Autodesk Inventor part; units mm, degrees
ref_plane "YZ Plane" through (0, 0, 0) normal (1, 0, 0) x (0, 1, 0)
ref_plane "XZ Plane" through (0, 0, 0) normal (0, 1, 0) x (-1, 0, 0)
ref_plane "XY Plane" through (0, 0, 0) normal (0, 0, 1) x (1, 0, 0)
sketch "Sketch1" plane through (0, 0, 0) normal (0, 0, 1) x (1, 0, 0)
  line L0 (0, 0) -> (120, 0)
  line L1 (120, 0) -> (120, 80)
  line L2 (120, 80) -> (0, 80)
  line L3 (0, 80) -> (0, 0)
  dimension "d0" = 120
  dimension "d1" = 80
extrude "Extrusion1" add sketch "Sketch1" along normal blind 6
sketch "Sketch2" plane through (0, 0, 6) normal (0, 0, 1) x (1, 0, 0)
  line L0 (0, 0) -> (120, 0)
  line L1 (120, 0) -> (120, 80)
  line L2 (120, 80) -> (0, 80)
  line L3 (0, 80) -> (0, 0)
  line L4 (120, 0) -> (105.25, 0)
  line L5 (105.25, 0) -> (105.25, 6)
  line L6 (105.25, 6) -> (120, 6)
  line L7 (120, 6) -> (120, 0)
  line L8 (0, 0) -> (120, 0)
  line L9 (74.75, 0) -> (45.25, 0)
  line L10 (45.25, 0) -> (45.25, 6)
  line L11 (45.25, 6) -> (74.75, 6)
  line L12 (74.75, 6) -> (74.75, 0)
  line L13 (14.75, 0) -> (0, 0)
  line L14 (0, 0) -> (0, 6)
  line L15 (0, 6) -> (14.75, 6)
  line L16 (14.75, 6) -> (14.75, 0)
  line L17 (120, 80) -> (105.25, 80)
  line L18 (105.25, 80) -> (105.25, 74)
  line L19 (105.25, 74) -> (120, 74)
  line L20 (120, 74) -> (120, 80)
  line L21 (120, 80) -> (0, 80)
  line L22 (74.75, 80) -> (45.25, 80)
  line L23 (45.25, 80) -> (45.25, 74)
  line L24 (45.25, 74) -> (74.75, 74)
  line L25 (74.75, 74) -> (74.75, 80)
  line L26 (14.75, 80) -> (0, 80)
  line L27 (0, 80) -> (0, 74)
  line L28 (0, 74) -> (14.75, 74)
  line L29 (14.75, 74) -> (14.75, 80)
  line L30 (60, -24.5918) -> (60, 107.6161)
  line L31 (0, 80) -> (0, 0)
  dimension "d4" = 6
  dimension "d5" = 6
  dimension "d6" = 14.75
  dimension "d7" = 14.75
  dimension "d8" = 29.5
  dimension "d18" = 60
  dimension "d19" = 14.75
extrude "Extrusion2" cut sketch "Sketch2" against normal up to next contours L3 L15 L16 L0 | L10 L11 L30 L0 | L3 L2 L29 L28 | L30 L11 L12 L0 | L5 L6 L1 L0 | L30 L2 L25 L24 | L24 L23 L2 L30 | L19 L18 L2 L1
sketch "Sketch3" plane through (0, 0, 6) normal (0, 0, 1) x (1, 0, 0)
  circle A0 centre (80, 40) radius 4.6
  line L0 (74.75, 0) -> (105.25, 0)
  line L1 (120, 6) -> (120, 74)
  point P0 (0, 0)
  dimension "d13" = 9.2
  dimension "d14" = 40
  dimension "d15" = 40
extrude "Extrusion3" cut sketch "Sketch3" against normal up to next
sketch "Sketch4" plane through (0, 0, 6) normal (0, 0, 1) x (1, 0, 0)
  circle A0 centre (80, 40) radius 4.6
  line L0 (74.75, 6) -> (74.75, 0)
  line L1 (74.75, 0) -> (105.25, 0)
  line L2 (105.25, 0) -> (105.25, 6)
  line L3 (105.25, 6) -> (120, 6)
  line L4 (120, 6) -> (120, 74)
  line L5 (120, 74) -> (105.25, 74)
  line L6 (105.25, 74) -> (105.25, 80)
  line L7 (105.25, 80) -> (74.75, 80)
  line L8 (74.75, 80) -> (74.75, 74)
  line L9 (74.75, 74) -> (45.25, 74)
  line L10 (45.25, 74) -> (45.25, 80)
  line L11 (45.25, 80) -> (14.75, 80)
  line L12 (14.75, 80) -> (14.75, 74)
  line L13 (14.75, 74) -> (0, 74)
  line L14 (0, 74) -> (0, 6)
  line L15 (0, 6) -> (14.75, 6)
  line L16 (14.75, 6) -> (14.75, 0)
  line L17 (14.75, 0) -> (45.25, 0)
  line L18 (45.25, 0) -> (45.25, 6)
  line L19 (45.25, 6) -> (74.75, 6)
  circle A1 centre (80, 40) radius 14.125
  circle A2 centre (97.5, 40) radius 1.5
  circle A3 centre (74.5, 57) radius 1.5
  circle A4 centre (74.5, 23) radius 1.5
  circle A5 centre (35.064, 64.1) radius 1.5
  circle A6 centre (35.064, 15.9) radius 1.5
  line L20 (80, 40) -> (97.5, 40) construction
  circle A7 centre (10, 66.125) radius 2.3
  circle A8 centre (10, 51.125) radius 2.3
  circle A9 centre (10, 13.875) radius 2.3
  circle A10 centre (10, 28.875) radius 2.3
  circle A11 centre (110, 66.125) radius 2.3
  circle A12 centre (110, 51.125) radius 2.3
  circle A13 centre (110, 13.875) radius 2.3
  circle A14 centre (110, 28.875) radius 2.3
  line L21 (10, 66.125) -> (110, 66.125) construction
  line L22 (110, 66.125) -> (110, 13.875) construction
  line L23 (110, 13.875) -> (10, 13.875) construction
  line L24 (10, 13.875) -> (10, 66.125) construction
  circle A15 centre (10, 61.125) radius 2.3
  circle A16 centre (10, 54.125) radius 2.3
  circle A17 centre (10, 69.125) radius 2.3
  circle A18 centre (10, 46.525) radius 2.3
  circle A19 centre (10, 33.475) radius 2.3
  circle A20 centre (10, 25.875) radius 2.3
  circle A21 centre (10, 18.475) radius 2.3
  circle A22 centre (10, 10.875) radius 2.3
  circle A23 centre (110, 69.125) radius 2.3
  circle A24 centre (110, 61.525) radius 2.3
  circle A25 centre (110, 54.125) radius 2.3
  circle A26 centre (110, 46.525) radius 2.3
  circle A27 centre (110, 33.475) radius 2.3
  circle A28 centre (110, 25.875) radius 2.3
  circle A29 centre (110, 18.475) radius 2.3
  circle A30 centre (110, 10.875) radius 2.3
  line L25 (7.7, 69.125) -> (7.7, 61.125)
  line L26 (12.3, 61.125) -> (12.3, 69.125)
  line L27 (7.7, 54.125) -> (7.7, 46.525)
  line L28 (12.3, 46.525) -> (12.3, 54.125)
  line L29 (7.7, 10.875) -> (7.7, 18.475)
  line L30 (7.7, 25.875) -> (7.7, 33.475)
  line L31 (12.3, 33.475) -> (12.3, 25.875)
  line L32 (12.3, 18.475) -> (12.3, 10.875)
  line L33 (112.3, 61.525) -> (112.3, 69.125)
  line L34 (107.7, 69.125) -> (107.7, 61.525)
  line L35 (107.7, 54.125) -> (107.7, 46.525)
  line L36 (112.3, 46.525) -> (112.3, 54.125)
  line L37 (107.7, 33.475) -> (107.7, 25.875)
  line L38 (107.7, 18.475) -> (107.7, 10.875)
  line L39 (112.3, 10.875) -> (112.3, 18.475)
  line L40 (112.3, 25.875) -> (112.3, 33.475)
  point P0 (0, 0)
  dimension "d20" = 28.25
  dimension "d21" = 3
  dimension "d22" = 3
  dimension "d23" = 3
  dimension "d24" = 3
  dimension "d25" = 3
  dimension "d26" = 17.5
  dimension "d27" = 5.5
  dimension "d28" = 5.5
  dimension "d29" = 34
  dimension "d30" = 17
  dimension "d31" = 48.2
  dimension "d32" = 24.1
  dimension "d33" = 44.936
  dimension "d34" = 44.936
  dimension "d37" = 10
  dimension "d38" = 10
  dimension "d39" = 4.6
  dimension "d40" = 4.6
  dimension "d41" = 4.6
  dimension "d42" = 4.6
  dimension "d43" = 4.6
  dimension "d44" = 4.6
  dimension "d45" = 4.6
  dimension "d46" = 4.6
  dimension "d47" = 13.875
  dimension "d48" = 13.875
  dimension "d49" = 15
  dimension "d50" = 15
  dimension "d51" = 15
  dimension "d52" = 15
  dimension "d53" = 4.6
  dimension "d54" = 4.6
  dimension "d56" = 3
  dimension "d57" = 5
  dimension "d58" = 4.6
  dimension "d59" = 3
  dimension "d60" = 4.6
  dimension "d61" = 4.6
  dimension "d62" = 4.6
  dimension "d63" = 4.6
  dimension "d64" = 4.6
  dimension "d65" = 3
  dimension "d66" = 3
  dimension "d67" = 4.6
  dimension "d68" = 4.6
  dimension "d69" = 4.6
  dimension "d70" = 4.6
  dimension "d71" = 4.6
  dimension "d72" = 4.6
  dimension "d73" = 4.6
  dimension "d74" = 4.6
  dimension "d75" = 3
  dimension "d76" = 3
  dimension "d77" = 3
  dimension "d78" = 3
extrude "Extrusion4" cut sketch "Sketch4" against normal blind 10 contours A1 | A2 | A3 | A4 | A5 | A6
extrude "Extrusion5" cut sketch "Sketch4" against normal blind 10 contours A7 A17 | L26 A15 L25 A7 | A7 A17 L26 | A17 A7 | A7 A17 | L25 A17 A7 | A15 | A8 A16 | L28 A18 A8 | A8 A16 L28 | A16 A8 | A8 A16 | A18 L27 A8 | A18 | A8 L27 A16 | A9 A22 | L32 A22 A9 | A9 A21 L32 | A9 L29 A21 | A21 | A22 A9 | A9 A22 | A9 A22 L29 | A10 A20 | L31 A20 A10 | A10 A19 L31 | A10 L30 A19 | A19 | A20 A10 | A10 A20 | A10 A20 L30 | A11 A23 | L33 A24 A11 | A11 A23 L33 | A23 A11 | A11 A23 | A24 L34 A11 | A24 | A11 L34 A23 | A12 A25 | L36 A26 A12 | A12 A25 L36 | A25 A12 | A12 A25 | A26 L35 A12 | A26 | A12 L35 A25 | A13 A30 | L39 A30 A13 | A13 A29 L39 | A13 L38 A29 | A29 | A30 A13 | A13 A30 | A13 A30 L38 | A14 A28 | L40 A28 A14 | A14 A27 L40 | A14 L37 A27 | A27 | A28 A14 | A14 A28 | A14 A28 L37
sketch "Sketch6" plane through (0, 0, 6) normal (0, 0, 1) x (1, 0, 0)
  line L0 (107.7, 25.875) -> (107.7, 33.475)
  arc A0 (112.3, 33.475) -> (107.7, 33.475) centre (110, 33.475) ccw
  line L1 (112.3, 33.475) -> (112.3, 25.875)
  arc A1 (107.7, 25.875) -> (112.3, 25.875) centre (110, 25.875) ccw
  line L2 (7.7, 25.875) -> (7.7, 33.475)
  arc A2 (12.3, 33.475) -> (7.7, 33.475) centre (10, 33.475) ccw
  line L3 (12.3, 33.475) -> (12.3, 25.875)
  arc A3 (7.7, 25.875) -> (12.3, 25.875) centre (10, 25.875) ccw
  line L4 (12.3, 54.125) -> (12.3, 46.525)
  arc A4 (7.7, 46.525) -> (12.3, 46.525) centre (10, 46.525) ccw
  line L5 (7.7, 46.525) -> (7.7, 54.125)
  arc A5 (12.3, 54.125) -> (7.7, 54.125) centre (10, 54.125) ccw
  line L6 (7.7, 10.875) -> (7.7, 18.475)
  arc A6 (12.3, 18.475) -> (7.7, 18.475) centre (10, 18.475) ccw
  line L7 (12.3, 18.475) -> (12.3, 10.875)
  arc A7 (7.7, 10.875) -> (12.3, 10.875) centre (10, 10.875) ccw
  line L8 (107.7, 61.525) -> (107.7, 69.125)
  arc A8 (112.3, 69.125) -> (107.7, 69.125) centre (110, 69.125) ccw
  line L9 (112.3, 69.125) -> (112.3, 61.525)
  arc A9 (107.7, 61.525) -> (112.3, 61.525) centre (110, 61.525) ccw
  line L10 (112.3, 18.475) -> (112.3, 10.875)
  arc A10 (107.7, 10.875) -> (112.3, 10.875) centre (110, 10.875) ccw
  line L11 (107.7, 10.875) -> (107.7, 18.475)
  arc A11 (112.3, 18.475) -> (107.7, 18.475) centre (110, 18.475) ccw
  line L12 (7.7, 61.125) -> (7.7, 69.125)
  arc A12 (12.3, 69.125) -> (7.7, 69.125) centre (10, 69.125) ccw
  line L13 (12.3, 69.125) -> (12.3, 61.125)
  arc A13 (7.7, 61.125) -> (12.3, 61.125) centre (10, 61.125) ccw
  line L14 (112.3, 54.125) -> (112.3, 46.525)
  arc A14 (107.7, 46.525) -> (112.3, 46.525) centre (110, 46.525) ccw
  line L15 (107.7, 46.525) -> (107.7, 54.125)
  arc A15 (112.3, 54.125) -> (107.7, 54.125) centre (110, 54.125) ccw
  circle A16 centre (80, 40) radius 14.125
  circle A17 centre (35.064, 64.1) radius 1.5
  circle A18 centre (74.5, 57) radius 1.5
  circle A19 centre (97.5, 40) radius 1.5
  circle A20 centre (74.5, 23) radius 1.5
  circle A21 centre (35.064, 15.9) radius 1.5
  line L16 (74.75, 6) -> (74.75, 0)
  line L17 (74.75, 0) -> (105.25, 0)
  line L18 (105.25, 0) -> (105.25, 6)
  line L19 (105.25, 6) -> (120, 6)
  line L20 (120, 6) -> (120, 74)
  line L21 (120, 74) -> (105.25, 74)
  line L22 (105.25, 74) -> (105.25, 80)
  line L23 (105.25, 80) -> (74.75, 80)
  line L24 (74.75, 80) -> (74.75, 74)
  line L25 (74.75, 74) -> (45.25, 74)
  line L26 (45.25, 74) -> (45.25, 80)
  line L27 (45.25, 80) -> (14.75, 80)
  line L28 (14.75, 80) -> (14.75, 74)
  line L29 (14.75, 74) -> (0, 74)
  line L30 (0, 74) -> (0, 6)
  line L31 (0, 6) -> (14.75, 6)
  line L32 (14.75, 6) -> (14.75, 0)
  line L33 (14.75, 0) -> (45.25, 0)
  line L34 (45.25, 0) -> (45.25, 6)
  line L35 (45.25, 6) -> (74.75, 6)
  circle A22 centre (97.765, 15.9) radius 1.5
  circle A23 centre (97.765, 64.1) radius 1.5
  point P0 (0, 0)
  dimension "d94" = 62.701
  dimension "d95" = 15.9
  dimension "d96" = 15.9
  dimension "d97" = 3
  dimension "d98" = 62.701
  dimension "d99" = 15.9
  dimension "d100" = 3
extrude "Extrusion7" cut sketch "Sketch6" against normal blind 10 contours A22 | A23
equation "\"d22\" = d21"
equation "\"d23\" = d21"
equation "\"d24\" = d21"
equation "\"d25\" = d21"
equation "\"d30\" = 0.5 * d29"
equation "\"d32\" = 0.5 * d31"
equation "\"d34\" = d33"
equation "\"d39\" = d64"
equation "\"d40\" = d64"
equation "\"d41\" = d64"
equation "\"d42\" = d64"
equation "\"d43\" = d74"
equation "\"d44\" = d74"
equation "\"d45\" = d74"
equation "\"d46\" = d74"
equation "\"d48\" = d47"
equation "\"d53\" = d64"
equation "\"d54\" = d64"
equation "\"d58\" = d64"
equation "\"d60\" = d64"
equation "\"d61\" = d64"
equation "\"d62\" = d64"
equation "\"d63\" = d64"
equation "\"d67\" = d74"
equation "\"d68\" = d74"
equation "\"d69\" = d74"
equation "\"d70\" = d74"
equation "\"d71\" = d74"
equation "\"d72\" = d74"
equation "\"d73\" = d74"
equation "\"d96\" = d95"
equation "\"d98\" = d94"
equation "\"d99\" = d96"
properties part number "bottom"
Design review of the part built by this model. Coordinates are the model's own, in mm. A direction names the side the tool comes from. Coordinates: 2 decimals unless noted, no trailing zeros. Order: outer loops, then holes, each group sorted by start corner. A loop starts at its lowest first (then second) coordinate and runs counter-clockwise, first axis right, second up.
Item 1: Take a section at A-A, the plane x = 10. Write out the cut boundary in (y, z) (3 decimals).
Item 2: Take a section at B-B, the plane y = 40. Write out the cut boundary in (x, z) (3 decimals), then the cut area to 4 significant figures.
Item 3: For faces 4 (the flat face through (74.75, 77, 3)), 5 (the flat face through (7, 74, 3)), 6 (the flat face through (120, 40, 3)), 7 (the flat face through (112.3, 30, 3)), 8 (the flat face through (14.75, 3, 3)), list the 3-axis set-ups (+Z, -Z, +X, -X, +Y, -Y) from which the entire face can be reached by the end or side of a thin tool; tool diameter is ignored.
Item 4: For pin 1 Ø3 at (x, z) = (12, 5.5) entering from -Y, flat-tipped, find the tip position at first contact; note if it passes through.
Item 5: Take a section at C-C, the plane x = 80. Write out the cut boundary in (y, z) (3 decimals), then the cut area to 4 significant figures.
Item 6: Take a section at D-D, the plane y = 15.9. Write out the cut boundary in (x, z) (3 decimals), then the cut area to 3 significant figures.
Item 7: The part is to be moulded in two halves that separate along X. For faces 1 (the flat face through (14.75, 77, 3)), 2 (the flat face through (30, 80, 3)), 3 (the flat face through (45.25, 3, 3)), say which applies: pulls with the +X half, pulls with the -X half, needs draft (parallel to the pull), parting line crosses it, or undercut.
Item 8: For line 1 (X direction, y = 62.5, z = 2.5); line 2 (X direction, y = 64.1, z = 4.55) (3 decimals); line 3 (Y direction, x = 109, z = 4.4), list the stretches that pass through material, from the lowest coordinate up.
The answers:
1. outline: (6, 0) - (8.575, 0) - (8.575, 6) - (6, 6) - close; (20.775, 0) - (23.575, 0) - (23.575, 6) - (20.775, 6) - close; (35.775, 0) - (44.225, 0) - (44.225, 6) - (35.775, 6) - close; (56.425, 0) - (58.825, 0) - (58.825, 6) - (56.425, 6) - close; (71.425, 0) - (74, 0) - (74, 6) - (71.425, 6) - close
2. outline: (0, 0) - (65.875, 0) - (65.875, 6) - (0, 6) - close; (94.125, 0) - (96, 0) - (96, 6) - (94.125, 6) - close; (99, 0) - (120, 0) - (120, 6) - (99, 6) - close
2. area: 532.5 mm2
3. face 4: +Z, -Z, +Y
3. face 5: +Z, -Z, -X, +Y
3. face 6: +Z, -Z, +X, +Y, -Y
3. face 7: +Z, -Z
3. face 8: +Z, -Z, -X, -Y
4. pin 1: stops at y = 6
5. outline: (0, 0) - (25.875, 0) - (25.875, 6) - (0, 6) - close; (54.125, 0) - (80, 0) - (80, 6) - (54.125, 6) - close
5. area: 310.5 mm2
6. outline: (0, 0) - (7.7, 0) - (7.7, 6) - (0, 6) - close; (12.3, 0) - (33.564, 0) - (33.564, 6) - (12.3, 6) - close; (36.564, 0) - (96.265, 0) - (96.265, 6) - (36.564, 6) - close; (99.265, 0) - (107.7, 0) - (107.7, 6) - (99.265, 6) - close; (112.3, 0) - (120, 0) - (120, 6) - (112.3, 6) - close
6. area: 629 mm2
7. face 1: pulls with the -X half
7. face 2: needs draft
7. face 3: undercut
8. line 1: x = 0 to 7.7, 12.3 to 107.7, 112.3 to 120
8. line 2: x = 0 to 7.7, 12.3 to 33.564, 36.564 to 96.265, 99.265 to 107.7, 112.3 to 120
8. line 3: y = 6 to 8.8, 20.55 to 23.8, 35.55 to 44.45, 56.2 to 59.45, 71.2 to 74
